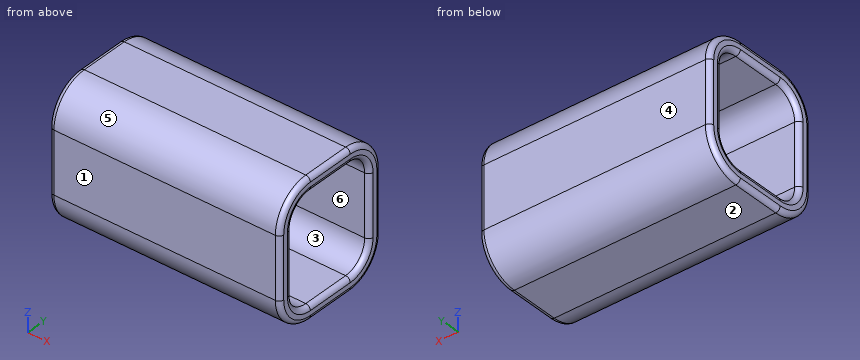
```python
from build123d import *

# Parameters (mm, degrees)
F1_DEPTH = 254
F2_R     = 5.08


with BuildPart() as f1:
    # F0 (on Right) → F1 (new body)
    with BuildSketch(Plane.YZ):
        with BuildLine():
            Line((72.400342, -31.400991), (72.400342, 36.261361))
            ThreePointArc((72.400342, 36.261361), (60.497162, 64.99818), (31.760342, 76.901361))
            Line((31.760342, 76.901361), (-21.520933, 76.901361))
            ThreePointArc((-21.520933, 76.901361), (-50.257752, 64.99818), (-62.160933, 36.261361))
            Line((-62.160933, 36.261361), (-62.160933, -31.400991))
            ThreePointArc((-62.160933, -31.400991), (-50.257752, -60.137811), (-21.520933, -72.040991))
            Line((-21.520933, -72.040991), (31.760342, -72.040991))
            ThreePointArc((31.760342, -72.040991), (60.497162, -60.137811), (72.400342, -31.400991))
        make_face()
        with BuildLine():
            ThreePointArc((-46.920933, 36.261361), (-39.481445, 54.221873), (-21.520933, 61.661361))
            Line((-21.520933, 61.661361), (31.760342, 61.661361))
            ThreePointArc((31.760342, 61.661361), (49.720854, 54.221873), (57.160342, 36.261361))
            Line((57.160342, 36.261361), (57.160342, -31.400991))
            ThreePointArc((57.160342, -31.400991), (49.720854, -49.361504), (31.760342, -56.800991))
            Line((31.760342, -56.800991), (-21.520933, -56.800991))
            ThreePointArc((-21.520933, -56.800991), (-39.481445, -49.361504), (-46.920933, -31.400991))
            Line((-46.920933, -31.400991), (-46.920933, 36.261361))
        make_face(mode=Mode.SUBTRACT)
    extrude(amount=F1_DEPTH)

    # F2
    f2_edges = [f1.edges().sort_by_distance(p)[0] for p in [
        (254, 5.119705, 61.661361),
        (254, 5.119705, 76.901361),
        (254, 60.497162, 64.99818),
        (254, 49.720854, 54.221873),
        (254, 57.160342, 2.430185),
        (254, 60.497162, -60.137811),
        (254, 49.720854, -49.361504),
        (254, 72.400342, 2.430185),
        (254, 5.119705, -56.800991),
        (254, 5.119705, -72.040991),
        (254, -39.481445, -49.361504),
        (254, -50.257752, -60.137811),
        (254, -62.160933, 2.430185),
        (254, -46.920933, 2.430185),
        (254, -50.257752, 64.99818),
        (254, -39.481445, 54.221873),
        (0, 72.400342, 2.430185),
        (0, 57.160342, 2.430185),
        (0, 60.497162, 64.99818),
        (0, 5.119705, 61.661361),
        (0, 49.720854, 54.221873),
        (0, 5.119705, 76.901361),
        (0, -50.257752, 64.99818),
        (0, -39.481445, 54.221873),
        (0, -46.920933, 2.430185),
        (0, -62.160933, 2.430185),
        (0, -50.257752, -60.137811),
        (0, -39.481445, -49.361504),
        (0, 5.119705, -72.040991),
        (0, 5.119705, -56.800991),
        (0, 60.497162, -60.137811),
        (0, 49.720854, -49.361504),
    ]]
    fillet(f2_edges, radius=F2_R)


solid = f1.part
```
Check sheet for the modelled part. Datum: model origin and axes. Units: mm. Face numbers are marked on the shaded views. A direction names the side the tool comes from. Coordinates: 2 decimals unless noted, no trailing zeros. Order: outer loops, then holes, each group sorted by start corner. A loop starts at its lowest first (then second) coordinate and runs counter-clockwise, first axis right, second up. Notation, with made-up numbers: (75, 14.25) -> (84, 14.25) arc R17 cw to (84, 24.25) -> close; hole circle Ø3 at (19.5, 27.5). An arc over 180 degrees is marked (long way). Write item = value, one per line. Start each with the question number.
1) Cross-section at B-B (x = 33.5). Enter the section's corners in (y, z).
2) Cross-section at C-C (y = 18.5). Enter the section's corners in (x, z), then the cut area to 3 significant figures.
3) Mould release check, pull along Y, two halves, no side actions. Record for the marked faces 1, 2, 3 and 4: +Y half, -Y half, draft (parallel to the pull), parting line (faces both ways), or undercut.
4) Go/stop test with flat-tipped pins: P1, Ø2, axis at y = -36.5, z = 58.5, coming from the -X side; P2, Ø2, axis at y = 57.5, z = 29, coming from the +X side. Record where each tip stops, or that it passes through.
5) Cross-section at A-A (z = 27). Enter the section's corners in (x, y), then the cut area to 3 significant figures.
6) Access from +Z, -Z, +X, -X, +Y, -Y to the whole of each face (thin tool, end or side, straight path). Record for the marked faces 5 and 6.
7) Material ranges on L1, parallel to Y at x = 141.5, z = -33; L2, parallel to Y at x = 56.5, z = 35.5; L3, parallel to Z at x = 34, y = -17, recorded low to high.
Ans:
q1.outline = (-62.16, -31.4) arc R40.64 ccw to (-21.52, -72.04) -> (31.76, -72.04) arc R40.64 ccw to (72.4, -31.4) -> (72.4, 36.26) arc R40.64 ccw to (31.76, 76.9) -> (-21.52, 76.9) arc R40.64 ccw to (-62.16, 36.26) -> close; hole (-46.92, -31.4) arc R25.4 ccw to (-21.52, -56.8) -> (31.76, -56.8) arc R25.4 ccw to (57.16, -31.4) -> (57.16, 36.26) arc R25.4 ccw to (31.76, 61.66) -> (-21.52, 61.66) arc R25.4 ccw to (-46.92, 36.26) -> close
q2.outline = (0, -66.96) arc R5.08 ccw to (5.08, -72.04) -> (248.92, -72.04) arc R5.08 ccw to (254, -66.96) -> (254, -61.88) arc R5.08 ccw to (248.92, -56.8) -> (5.08, -56.8) arc R5.08 ccw to (0, -61.88) -> close; (0, 66.74) arc R5.08 ccw to (5.08, 61.66) -> (248.92, 61.66) arc R5.08 ccw to (254, 66.74) -> (254, 71.82) arc R5.08 ccw to (248.92, 76.9) -> (5.08, 76.9) arc R5.08 ccw to (0, 71.82) -> close
q2.area = 7,700 mm²
q3.face_1 = -Y half
q3.face_2 = draft
q3.face_3 = undercut
q3.face_4 = +Y half
q4.P1 = 0.76
q4.P2 = 252.36
q5.outline = (0, -57.08) arc R5.08 ccw to (5.08, -62.16) -> (248.92, -62.16) arc R5.08 ccw to (254, -57.08) -> (254, -52) arc R5.08 ccw to (248.92, -46.92) -> (5.08, -46.92) arc R5.08 ccw to (0, -52) -> close; (0, 62.24) arc R5.08 ccw to (5.08, 57.16) -> (248.92, 57.16) arc R5.08 ccw to (254, 62.24) -> (254, 67.32) arc R5.08 ccw to (248.92, 72.4) -> (5.08, 72.4) arc R5.08 ccw to (0, 67.32) -> close
q5.area = 7,700 mm²
q6.face_5 = +Z, +X, -X, -Y
q6.face_6 = +X, -X
q7.L1 = -62.13 to -46.87, 57.11 to 72.37
q7.L2 = -62.16 to -46.92, 57.16 to 72.4
q7.L3 = -72.04 to -56.8, 61.66 to 76.9
